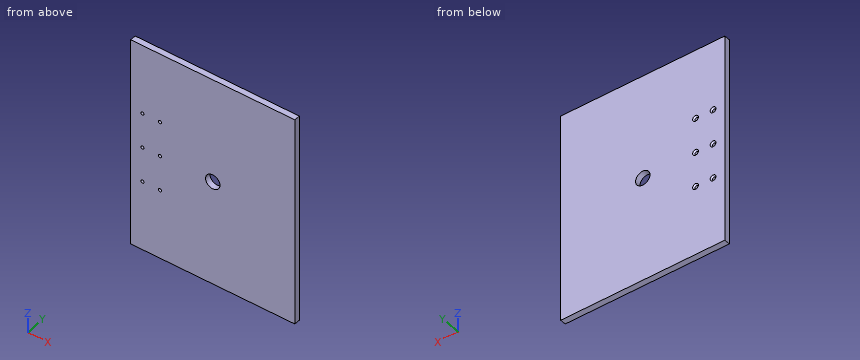
```python
from build123d import *

# Parameters (mm, degrees)
SKETCH1_W                                            = 177.8
SKETCH1_H                                            = 228.6
BOSS_EXTRUDE1_DEPTH                                  = 6.35
CUT_EXTRUDE1_REACH                                   = 213.465
SKETCH6_R                                            = 7.810000001
THREADED_CSK_FOR_M3_10_FLAT_HEAD_MACHINE_D           = 3.4
THREADED_CSK_FOR_M3_10_FLAT_HEAD_MACHINE_CSINK_D     = 6.3
THREADED_CSK_FOR_M3_10_FLAT_HEAD_MACHINE_CSINK_ANGLE = 90


with BuildPart() as part:
    # Sketch1 → Boss-Extrude1 (new body)
    with BuildSketch(Plane(origin=(0, 0, 0), x_dir=(1, 0, 0), z_dir=(0, 1, 0))):
        with Locations((88.9, 0)):
            Rectangle(SKETCH1_W, SKETCH1_H)
    extrude(amount=BOSS_EXTRUDE1_DEPTH)

    # Sketch6 → Cut-Extrude1 (cut, up to next)
    with BuildSketch(Plane(origin=(0, 6.35, 0), x_dir=(1, 0, 0), z_dir=(0, 1, 0)), mode=Mode.PRIVATE) as cut_extrude1_sk1:
        with Locations(Location((88.9, 0, 0), (0, 0, 270))):
            Circle(SKETCH6_R)
    cut_extrude1_tool1 = extrude(cut_extrude1_sk1.sketch, amount=-CUT_EXTRUDE1_REACH, mode=Mode.PRIVATE) & part.part
    add(cut_extrude1_tool1.solids().sort_by_distance((88.9, 6.35, 0))[0], mode=Mode.SUBTRACT)

    # Threaded CSK for M3-10 Flat Head Machine Screw1 (through all)
    with Locations(Plane(origin=(0, 6.35, 0), x_dir=(-1, 0, 0), z_dir=(0, 1, 0))):
        with Locations((-12.7, 0), (-12.7, 38.1), (-31.75, 38.1), (-12.7, -38.1), (-31.75, -38.1), (-31.75, 0)):
            CounterSinkHole(THREADED_CSK_FOR_M3_10_FLAT_HEAD_MACHINE_D / 2, THREADED_CSK_FOR_M3_10_FLAT_HEAD_MACHINE_CSINK_D / 2, counter_sink_angle=THREADED_CSK_FOR_M3_10_FLAT_HEAD_MACHINE_CSINK_ANGLE)


solid = part.part
```
Can you work these out from the model? Positions are in its coordinate system, mm. Coordinates: 2 decimals unless noted, no trailing zeros. Loops run counter-clockwise (first coordinate to the right, second up) from the corner with the lowest first, then second, coordinate; pieces in that order, holes last. Notation, with made-up numbers: (7, 29) -> (65, 29) arc R17 ccw to (65, 51) -> close; hole circle Ø6 at (-23, 78). An arc over 180 degrees is marked (long way). Put each result on its own line as item: value. Start each with the question number.
Q1. I'm going to push flat-ended pins straight in: P1, Ø4.5, axis at x = 12.7, z = -38.1, coming from the +Y side; P2, Ø5.5, axis at x = 31.75, z = -38.1, coming from the +Y side. Where does each tip first touch, or does it pass through?
Q2. If I drill on line 1 (X direction, y = 2, z = -38.1); line 2 (Z direction, x = 31.75, y = 2.55); line 3 (X direction, y = 3.4, z = 0), over which ranges is the centre line in solid material (lowest first)? Write a range as [from, to].
Q3. I want a section at A-A (x = 88.9). Write out the boundary of the cut face in (y, z), plus the area to 3 significant figures.
Taken from the geometry:
1. P1: stops at y = 5.45
1. P2: stops at y = 5.95
2. line 1: x = [0, 11], [14.4, 30.05], [33.45, 177.8]
2. line 2: z = [-114.3, -39.8], [-36.4, -1.7], [1.7, 36.4], [39.8, 114.3]
2. line 3: x = [0, 11], [14.4, 30.05], [33.45, 81.09], [96.71, 177.8]
3. outline: (0, -114.3) -> (6.35, -114.3) -> (6.35, -7.81) -> (0, -7.81) -> close; (0, 7.81) -> (6.35, 7.81) -> (6.35, 114.3) -> (0, 114.3) -> close
3. area: 1,350 mm2
